```python
from build123d import *

# Parameters (mm, degrees)
F0_R     = 12.7
F1_DEPTH = 25.4
F2_R     = 12.7
F3_DEPTH = 50.8
F4_R     = 12.7


with BuildPart() as f1:
    # F0 (on Front) → F1 (new body)
    with BuildSketch(Plane.XZ):
        with BuildLine():
            Line((64.218075, -10.262585), (-23.134906, 48.871121))
            ThreePointArc((-23.134906, 48.871121), (-49.279468, 50.274275), (-62.773699, 27.837415))
            Line((-62.773699, 27.837415), (-62.773699, -22.962585))
            Line((-62.773699, -22.962585), (64.218075, -22.962585))
            Line((64.218075, -22.962585), (64.218075, -10.262585))
        make_face()
        with Locations((-37.373699, 27.837415)):
            Circle(F0_R, mode=Mode.SUBTRACT)
    extrude(amount=F1_DEPTH)

    # F2 (on Front) → F3 (join)
    with BuildSketch(Plane.XZ):
        with BuildLine():
            Line((-11.877737, -11.430001), (-11.877737, 28.269436))
            ThreePointArc((-11.877737, 28.269436), (-37.277737, 53.669436), (-62.677737, 28.269436))
            Line((-62.677737, 28.269436), (-62.1792, -11.430001))
            Line((-62.1792, -11.430001), (-62.1792, -22.529295))
            Line((-62.1792, -22.529295), (64.197391, -22.529295))
            Line((64.197391, -22.529295), (64.197391, -11.430001))
            Line((64.197391, -11.430001), (-11.877737, -11.430001))
        make_face()
        with Locations((-37.277737, 28.269436)):
            Circle(F2_R, mode=Mode.SUBTRACT)
    extrude(amount=F3_DEPTH)

    # F4
    f4_edges = [f1.edges().sort_by_distance(p)[0] for p in [
        (64.197391, -50.8, -16.979648),
    ]]
    fillet(f4_edges, radius=F4_R)


solid = f1.part
```
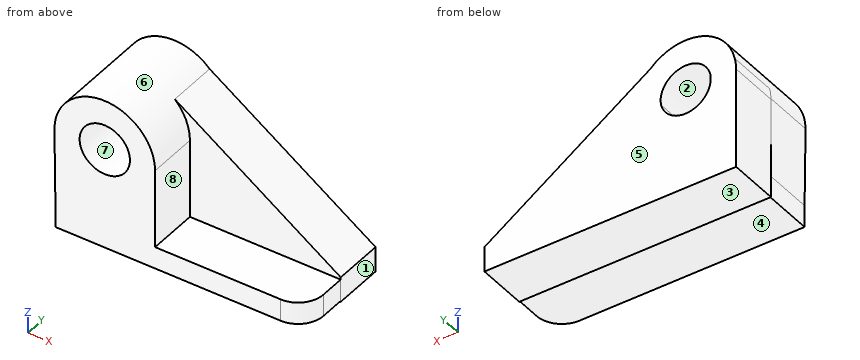
Work out the finished part from the listing and answer in its coordinate system (mm). Face numbers are marked on the shaded views. A direction names the side the tool comes from. Give positions to 0.01 mm unless a question says otherwise; leave off trailing zeros. Write each loop counter-clockwise with the first axis right and the second up, starting at its lowest first coordinate (ties: lowest second). Pieces come first, ordered by that corner, then holes.
(1) The part is cut by section D-D on z = 4.5. Write down the section's boundary in (x, y), plus the area to 3 significant figures.
Final values:
outline: (-62.77, -25.4) - (-62.38, -25.4) - (-62.38, -50.8) - (-11.88, -50.8) - (-11.88, -25.4) - (42.41, -25.4) - (42.41, 0) - (-62.77, 0) - close
area: 3,950 mm2
(2) Straight lines are drawn through the part: line 1 (Z direction, x = -38, y = -29.5); line 2 (Y direction, x = -9.5, z = 31.5); line 3 (X direction, y = -25, z = 25). For each, find the intervals that lie inside material, in ascending order.
Final values:
line 1: z = -22.53 to 15.59, 40.95 to 53.66
line 2: y = -25.4 to 0
line 3: x = -62.77 to -49.55, -25.01 to 12.13
(3) The part is cut by section C-C on x = 55.5. Write down the section's boundary in (y, z).
Final values:
outline: (-50.15, -22.53) - (-25.4, -22.53) - (-25.4, -22.96) - (0, -22.96) - (0, -4.36) - (-25.4, -4.36) - (-25.4, -11.43) - (-50.15, -11.43) - close
(4) Which of the six approach directions +Z, -Z, +X, -X, +Y, -Y give full straight-line access (tool end or side, diameter ignored) to the marked faces 4, 5, 6, 7 and 8?
Final values:
face 4: -Z, +X, -X, -Y
face 5: +Z, -Z, +X, -X, +Y
face 6: +Z, -Y
face 7: -Y
face 8: +Z, +X, -Y
(5) Flat-ended cylindrical pins translate along their axes: pin 1 Ø12.5 at (x, y) = (17, -40.5) entering from +Z; pin 2 Ø8 at (x, y) = (3.5, -16.5) entering from +Z; pin 3 Ø2 at (y, z) = (-26, 42) entering from -X. Find the tip coordinate at first contact, or state that the pin passes through.
Final values:
pin 1: stops at z = -11.43
pin 2: stops at z = 33.55
pin 3: stops at x = -59.26
(6) The mould has two halves that part along X. Classify the marked faces 1, 2 and 3: pulls with the +X half, pulls with the -X half, needs draft (parallel to the pull), parting line crosses it, or undercut.
Final values:
face 1: pulls with the +X half
face 2: undercut
face 3: needs draft
(7) The part is cut by section B-B on z = 22. Write down the section's boundary in (x, y), plus the area to 3 significant figures.
Final values:
outline: (-62.77, -25.4) - (-62.6, -25.4) - (-62.6, -50.8) - (-48.32, -50.8) - (-48.32, 0) - (-62.77, 0) - close; (-26.23, -50.8) - (-11.88, -50.8) - (-11.88, -25.4) - (16.56, -25.4) - (16.56, 0) - (-26.23, 0) - close
area: 2,180 mm2
(8) The part is cut by section A-A on y = -35. Write down the section's boundary in (x, z).
Final values:
outline: (-62.68, 28.27) - (-62.18, -11.43) - (-62.18, -22.53) - (64.2, -22.53) - (64.2, -11.43) - (-11.88, -11.43) - (-11.88, 28.27) arc R25.4 ccw to start; hole circle Ø25.4 at (-37.28, 28.27)
